The model under review builds one solid part; all positions refer to its coordinate system, in mm. Face numbers are marked on the shaded views. A direction names the side the tool comes from. Round coordinates to 2 decimals unless told otherwise and drop trailing zeros. Order: outer loops, then holes, each group sorted by start corner. A loop starts at its lowest first (then second) coordinate and runs counter-clockwise, first axis right, second up. Notation, with made-up numbers: (4, 87.5) -> (35, 87.5) arc R27 ccw to (35, 107.5) -> close; hole circle Ø1 at (-23.75, 77.5). An arc over 180 degrees is marked (long way). Use a Markdown table: item, result. Add a question column.
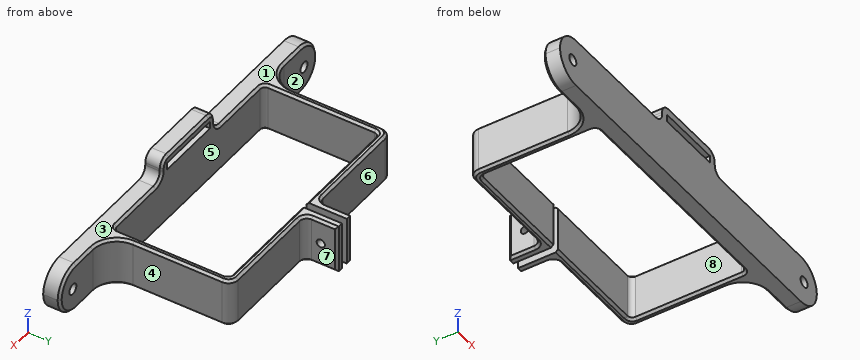
```python
from build123d import *

# Parameters (mm, degrees)
SKETCH1_W           = 161
SKETCH1_H           = 20
SKETCH1_R           = 2.2
BOSS_EXTRUDE1_DEPTH = 7
BOSS_EXTRUDE2_DEPTH = 20
SKETCH4_W           = 33
SKETCH4_H           = 9
SKETCH4_W_2         = 27
SKETCH4_H_2         = 3
BOSS_EXTRUDE3_DEPTH = 7
SKETCH5_R           = 1.7
CUT_EXTRUDE1_DEPTH  = 113.749988914
FILLET1_R           = 2
FILLET2_R           = 10
FILLET3_R           = 3
FILLET4_R           = 4
FILLET5_R           = 4
CHAMFER1_SIZE       = 1


with BuildPart() as part:
    # Sketch1 → Boss-Extrude1 (new body)
    with BuildSketch(Plane(origin=(0, 0, 0), x_dir=(1, 0, 0), z_dir=(0, 1, 0))):
        Rectangle(SKETCH1_W, SKETCH1_H)
        with Locations(Location((-72.5, 0, 0), (0, 0, 270))):
            Circle(SKETCH1_R, mode=Mode.SUBTRACT)
        with Locations(Location((72.5, 0, 0), (0, 0, 270))):
            Circle(SKETCH1_R, mode=Mode.SUBTRACT)
    extrude(amount=BOSS_EXTRUDE1_DEPTH)

    # Sketch2 → Boss-Extrude2 (add)
    with BuildSketch(Plane.XY.offset(10)):
        Polygon((47, 55), (47, 7), (50, 7), (50, 58), (4.5, 58), (4.5, 71.6), (1.5, 71.6), (1.5, 55), align=None)
        Polygon((-50, 58), (-50, 7), (-47, 7), (-47, 55), (-1.5, 55), (-1.5, 71.6), (-4.5, 71.6), (-4.5, 58), align=None)
    extrude(amount=-BOSS_EXTRUDE2_DEPTH)

    # Sketch4 → Boss-Extrude3 (add)
    with BuildSketch(Plane(origin=(0, 0, 0), x_dir=(1, 0, 0), z_dir=(0, 1, 0))):
        with Locations((0, -14.5)):
            Rectangle(SKETCH4_W, SKETCH4_H)
        with Locations((0, -14.5)):
            Rectangle(SKETCH4_W_2, SKETCH4_H_2, mode=Mode.SUBTRACT)
    extrude(amount=BOSS_EXTRUDE3_DEPTH)

    # Sketch5 → Cut-Extrude1 (cut, through all)
    with BuildSketch(Plane.ZY.offset(4.5)):
        with Locations(Location((0, 64.8, 0), (0, 0, 270))):
            Circle(SKETCH5_R)
    extrude(amount=-CUT_EXTRUDE1_DEPTH, mode=Mode.SUBTRACT)

    # Fillet1
    fillet1_edges = [part.edges().sort_by_distance(p)[0] for p in [
        (47, 55, 0),
        (47, 7, 0),
        (-47, 55, 0),
        (-47, 7, 0),
    ]]
    fillet(fillet1_edges, radius=FILLET1_R)

    # Fillet2
    fillet2_edges = [part.edges().sort_by_distance(p)[0] for p in [
        (50, 7, 0),
        (-50, 7, 0),
        (80.5, 3.5, 10),
        (-80.5, 3.5, 10),
        (-80.5, 3.5, -10),
        (80.5, 3.5, -10),
    ]]
    fillet(fillet2_edges, radius=FILLET2_R - 0.0001)  # a hair under: the kernel refuses the full size

    # Fillet3
    fillet3_edges = [part.edges().sort_by_distance(p)[0] for p in [
        (4.5, 58, 0),
        (-4.5, 58, 0),
    ]]
    fillet(fillet3_edges, radius=FILLET3_R)

    # Fillet4
    fillet4_edges = [part.edges().sort_by_distance(p)[0] for p in [
        (-16.5, 3.5, 10),
        (-16.5, 3.5, 19),
        (16.5, 3.5, 19),
        (16.5, 3.5, 10),
    ]]
    fillet(fillet4_edges, radius=FILLET4_R)

    # Fillet5
    fillet5_edges = [part.edges().sort_by_distance(p)[0] for p in [
        (50, 58, 0),
        (-50, 58, 0),
    ]]
    fillet(fillet5_edges, radius=FILLET5_R)

    # Chamfer1
    chamfer1_edges = [part.edges().sort_by_distance(p)[0] for p in [
        (46.414213562, 54.414213562, 10),
        (46.414213562, 54.414213562, -10),
        (46.414213562, 7.585786438, 10),
        (46.414213562, 7.585786438, -10),
        (-46.414213562, 7.585786438, 10),
        (-46.414213562, 7.585786438, -10),
        (-46.414213562, 54.414213562, 10),
        (-46.414213562, 54.414213562, -10),
        (65.25, 7, -10),
        (65.25, 7, 10),
        (77.571097101, 7, -7.071097101),
        (77.571097101, 7, 7.071097101),
        (50, 35.49995, 10),
        (-50, 35.49995, 10),
        (-65.25, 7, -10),
        (-65.25, 7, 10),
        (-77.571097101, 7, 7.071097101),
        (-77.571097101, 7, -7.071097101),
        (52.928902899, 9.928902899, 10),
        (52.928902899, 9.928902899, -10),
        (-52.928902899, 9.928902899, 10),
        (-52.928902899, 9.928902899, -10),
        (26.75, 58, -10),
        (4.5, 66.3, 10),
        (-4.5, 66.3, 10),
        (-26.75, 58, -10),
        (5.378679656, 58.878679656, 10),
        (5.378679656, 58.878679656, -10),
        (-5.378679656, 58.878679656, 10),
        (-5.378679656, 58.878679656, -10),
        (0, 7, 19),
        (-16.5, 7, 14.5),
        (32.75, 7, 10),
        (16.5, 7, 14.5),
        (15.328427125, 7, 17.828427125),
        (-15.328427125, 7, 17.828427125),
        (-17.671572875, 7, 11.171572875),
        (17.671572875, 7, 11.171572875),
        (50, 35.49995, -10),
        (26.75, 58, 10),
        (48.828427125, 56.828427125, 10),
        (-50, 35.49995, -10),
        (-48.828427125, 56.828427125, -10),
        (48.828427125, 56.828427125, -10),
        (-26.75, 58, 10),
        (-48.828427125, 56.828427125, 10),
        (4.5, 71.6, 0),
        (23.25, 55, -10),
        (4.5, 66.3, -10),
        (-4.5, 66.3, -10),
        (-4.5, 71.6, 0),
        (-23.25, 55, -10),
        (23.25, 55, 10),
        (47, 31, -10),
        (47, 31, 10),
        (0, 7, -10),
        (-32.75, 7, 10),
        (-47, 31, -10),
        (-47, 31, 10),
        (-23.25, 55, 10),
    ]]
    chamfer(chamfer1_edges, length=CHAMFER1_SIZE)


solid = part.part
```
Q1. For pin 1 (8 mm diameter, centred on x = -21.5, z = 3, fed in from +Y); pin 2 (4.5 mm diameter, centred on y = 64.8, z = 0, fed in from -X); pin 3 (14.5 mm diameter, centred on x = -74.5, z = -3.5, fed in from +Y); pin 4 (3 mm diameter, centred on x = 54, z = 13, fed in from -Y), all flat-tipped, find the tip position at first contact; note any pin that passes through.
Q2. Add section A-A, the plane y = 42. Give the boundary of the cut face in (x, z), then the cut area to 3 significant figures.
Q3. Add section B-B, the plane y = 64.8. Give the boundary of the cut face in (x, z), then the cut area to 3 significant figures.
Q4. Draft analysis for pull direction Y (two halves, no side actions). For the marked faces 6, 7 and 8, state which applies: released by +Y, released by -Y, zero draft, split by the parting line, or undercut.
Q5. To check wall thickness, follow line 1 along Y through (x, z) = (28, -3.75); line 2 along Z through (x, y) = (-2.5, 64.8); line 3 along X through (y, z) = (36.5, 0). State the ranges of each line that lie inside material, in increasing order.
Q6. Add section C-C, the plane x = -62. Give the boundary of the cut face in (y, z), then the cut area to 3 significant figures.
Q7. For the marked faces 1, 2, 3, 4 and 5, list the 3-axis set-ups (+Z, -Z, +X, -X, +Y, -Y) from which the entire face can be reached by the end or side of a thin tool; tool diameter is ignored.
Return value:
| question | item | result |
|---|---|---|
| 1 | pin 1 | y = 58 |
| 1 | pin 2 | x = -4.5 |
| 1 | pin 3 | y = 7 |
| 1 | pin 4 | through |
| 2 | outline | (-50, -9) -> (-49, -10) -> (-48, -10) -> (-47, -9) -> (-47, 9) -> (-48, 10) -> (-49, 10) -> (-50, 9) -> close; (47, -9) -> (48, -10) -> (49, -10) -> (50, -9) -> (50, 9) -> (49, 10) -> (48, 10) -> (47, 9) -> close |
| 2 | area | 116 mm² |
| 3 | outline | (-4.5, -9) -> (-3.5, -10) -> (-1.5, -10) -> (-1.5, -1.7) -> (-4.5, -1.7) -> close; (-4.5, 1.7) -> (-1.5, 1.7) -> (-1.5, 10) -> (-3.5, 10) -> (-4.5, 9) -> close; (1.5, -10) -> (3.5, -10) -> (4.5, -9) -> (4.5, -1.7) -> (1.5, -1.7) -> close; (1.5, 1.7) -> (4.5, 1.7) -> (4.5, 9) -> (3.5, 10) -> (1.5, 10) -> close |
| 3 | area | 97.6 mm² |
| 4 | face 6 | released by +Y |
| 4 | face 7 | zero draft |
| 4 | face 8 | undercut |
| 5 | line 1 | 0 to 7, 55 to 58 |
| 5 | line 2 | -10 to -1.7, 1.7 to 10 |
| 5 | line 3 | -50 to -47, 47 to 50 |
| 6 | outline | (0, -10) -> (6, -10) -> (7, -9) -> (7, 9) -> (6, 10) -> (0, 10) -> close |
| 6 | area | 139 mm² |
| 7 | face 1 | +Z, -X, +Y |
| 7 | face 2 | +Z, -Z, -X, +Y |
| 7 | face 3 | +Z, +X, +Y |
| 7 | face 4 | +Z, -Z, +X, +Y |
| 7 | face 5 | +Z, -Z |
